from build123d import *

# Parameters (mm, degrees)
SKETCH_1_W          = 86
SKETCH_1_H          = 45.2
EXTRUDE_1_DEPTH     = 7
SKETCH_4_R          = 12
SKETCH_4_W          = 6
SKETCH_4_H          = 5
EXTRUDE_2_DEPTH     = 10
SKETCH_5_R          = 16.25
CUT_EXTRUDE_1_DEPTH = 6
SKETCH_6_R          = 1.8
CUT_EXTRUDE_2_DEPTH = 20
SKETCH_7_R          = 3.5
CUT_EXTRUDE_3_DEPTH = 3.5


with BuildPart() as part:
    # 草图1 → 凸台-拉伸1 (new body)
    with BuildSketch(Plane(origin=(0, 0, 0), x_dir=(1, 0, 0), z_dir=(0, 1, 0))):
        with Locations((0, -3.4)):
            Rectangle(SKETCH_1_W, SKETCH_1_H)
    extrude(amount=EXTRUDE_1_DEPTH)

    # 草图4 → 凸台-拉伸2 (add)
    with BuildSketch(Plane(origin=(43, 0, 0), x_dir=(0, 0, -1), z_dir=(1, 0, 0))):
        with BuildLine():
            Line((19.2, 0), (-26, 0))
            Line((-26, 0), (-26, 33.5))
            ThreePointArc((-26, 33.5), (-3.4, 56.1), (19.2, 33.5))
            Line((19.2, 33.5), (19.2, 0))
        make_face()
        with Locations((-3.4, 33.5)):
            Circle(SKETCH_4_R, mode=Mode.SUBTRACT)
        with Locations((-20, 17.5)):
            Rectangle(SKETCH_4_W, SKETCH_4_H, mode=Mode.SUBTRACT)
        with Locations((13.2, 17.5)):
            Rectangle(SKETCH_4_W, SKETCH_4_H, mode=Mode.SUBTRACT)
    extrude(amount=-EXTRUDE_2_DEPTH)

    # 草图5 → 切除-拉伸1 (cut)
    with BuildSketch(Plane.ZY.offset(-33)):
        with Locations((3.4, 33.5)):
            Circle(SKETCH_5_R)
    extrude(amount=-CUT_EXTRUDE_1_DEPTH, mode=Mode.SUBTRACT)

    # 草图6 → 切除-拉伸2 (cut)
    with BuildSketch(Plane(origin=(0, 0, 0), x_dir=(1, 0, 0), z_dir=(0, 1, 0))):
        with Locations(Location((38, -20, 0), (0, 0, 90))):
            Circle(SKETCH_6_R)
        with Locations(Location((38.066919359, 12.870051801, 0), (0, 0, 90))):
            Circle(SKETCH_6_R)
    cut_extrude_2 = extrude(amount=CUT_EXTRUDE_2_DEPTH, mode=Mode.SUBTRACT)

    # 草图7 → 切除-拉伸3 (cut)
    with BuildSketch(Plane(origin=(0, 0, 0), x_dir=(1, 0, 0), z_dir=(0, 1, 0))):
        with Locations(Location((38, -20, 0), (0, 0, 270))):
            Circle(SKETCH_7_R)
        with Locations(Location((38, 13.2, 0), (0, 0, 90))):
            Circle(SKETCH_7_R)
    cut_extrude_3 = extrude(amount=CUT_EXTRUDE_3_DEPTH, mode=Mode.SUBTRACT)

    # 镜向1: 切除-拉伸2, 切除-拉伸3 across plane
    add(cut_extrude_2.mirror(Plane.ZY), mode=Mode.SUBTRACT)
    add(cut_extrude_3.mirror(Plane.ZY), mode=Mode.SUBTRACT)


solid = part.part
For this review, take the finished solid that the model builds, in its own axes (mm). A direction names the side the tool comes from. Round coordinates to 2 decimals unless told otherwise and drop trailing zeros. Order: outer loops, then holes, each group sorted by start corner. A loop starts at its lowest first (then second) coordinate and runs counter-clockwise, first axis right, second up. Notation, with made-up numbers: M -4,0 L 8,0 A6 ccw 8,11 Z; hole C 58.5,45.5 d8. An arc over 180 degrees is marked long. Write each question's results on one line, items separated by ' | '. Start each with the question number.
1. Add section A-A (y = 18.5). State the section outline as (x, z) points.
2. Tool access review of faces 1 (the face through (41.47, 1.73, 19.54)), 2 (the face through (33, 16, 3)), 3 (the face through (35.96, 49.61, 1.28)), 4 (the face through (38, 20, -13)): name each direction out of +Z, -Z, +X, -X, +Y, -Y from which nothing blocks a thin tool from reaching the whole face with its end or side.
3. Add section B-B (z = -3). State the section outline as (x, y) points.
4. Clearance check with flat-ended pins moving along their axes: pin 1 Ø6 at (x, z) = (38.07, -12.87) entering from +Y; pin 2 Ø2 at (x, z) = (-38.07, -12.87) entering from -Y; pin 3 Ø1 at (y, z) = (36.5, 16.5) entering from -X; pin 4 Ø2 at (x, z) = (-38.5, 18.5) entering from -Y. State where each tip first meets the part, or that it passes through.
5. Add section D-D (x = -29). State the section outline as (y, z) points.
6. Add section C-C (y = 39). State the section outline as (x, z) points.
7. To check wall thickness, follow L1, parallel to X at y = 1, z = 20; L2, parallel to Y at x = 41, z = 3; L3, parallel to Y at x = 37, z = 3. State the ranges of each line that lie inside material, in increasing order. Write a range as [from, to].
8. Draft analysis for pull direction Z (two halves, no side actions). For faces 5 (the face through (-6, 7, 3)), 6 (the face through (41.03, 43.62, -3.05)), 7 (the face through (38.07, 56.095, 3.897)), state which applies: pulls with the +Z half, pulls with the -Z half, needs draft (parallel to the pull), parting line crosses it, or undercut.
Output values:
1) outline: M 33,-19.2 L 43,-19.2 L 43,-16.2 L 33,-16.2 Z; M 33,-10.2 L 43,-10.2 L 43,17 L 33,17 L 33,9.65 L 39,9.65 L 39,-2.85 L 33,-2.85 Z; M 33,23 L 43,23 L 43,26 L 33,26 Z
2) face 1: -Y | face 2: +Z, -Z, -X, +Y | face 3: -X | face 4: +X, -X
3) outline: M -43,0 L 43,0 L 43,23.35 L 39,23.35 L 39,18.56 L 33,18.56 L 33,7 L -43,7 Z; M 33,48.44 L 39,48.44 L 39,43.65 L 43,43.65 L 43,55.17 L 33,55.17 Z
4) pin 1: y = 51.79 | pin 2: through | pin 3: x = 39 | pin 4: y = 3.5
5) outline: M 0,-19.2 L 7,-19.2 L 7,26 L 0,26 Z
6) outline: M 33,-18.52 L 43,-18.52 L 43,-7.27 L 39,-7.27 L 39,-11.89 L 33,-11.89 Z; M 33,18.69 L 39,18.69 L 39,14.07 L 43,14.07 L 43,25.32 L 33,25.32 Z
7) L1: [-43, -41.5], [-34.5, 34.5], [41.5, 43] | L2: [0, 21.51], [45.49, 56.1] | L3: [0, 17.25], [49.75, 56.1]
8) face 5: needs draft | face 6: undercut | face 7: parting line crosses it
